Source: CAD feature listing. Evaluate the final solid. Frame: model axes, mm. Coordinates: 2 decimals unless noted, no trailing zeros. Write each loop counter-clockwise with the first axis right and the second up, starting at its lowest first coordinate (ties: lowest second). Pieces come first, ordered by that corner, then holes. Notation, with made-up numbers: (66.25, -9) -> (117.25, -9) arc R12 cw to (117.25, 13) -> close; hole circle Ø8 at (10.25, 62). An arc over 180 degrees is marked (long way). Write item = value, one per line.
from build123d import *

# Parameters (mm, degrees)
SKETCH1_R           = 1.5
BOSS_EXTRUDE1_DEPTH = 2
CHAMFER1_SIZE       = 0.25


with BuildPart() as part:
    # Sketch1 → Boss-Extrude1 (new body)
    with BuildSketch(Plane(origin=(0, 0, 0), x_dir=(1, 0, 0), z_dir=(0, 1, 0))):
        Polygon((0, -3.464101615), (3, -1.732050808), (3, 1.732050808), (0, 3.464101615), (-3, 1.732050808), (-3, -1.732050808), align=None)
        Circle(SKETCH1_R, mode=Mode.SUBTRACT)
    extrude(amount=BOSS_EXTRUDE1_DEPTH)

    # Chamfer1
    chamfer1_edges = [part.edges().sort_by_distance(p)[0] for p in [
        (3, 2, 0),
        (1.5, 2, -2.598076211),
        (-1.5, 0, 0),
        (-1.5, 2, 0),
        (-1.5, 2, -2.598076211),
        (-3, 2, 0),
        (-1.5, 2, 2.598076211),
        (-3, 0, 0),
        (-1.5, 0, -2.598076211),
        (1.5, 0, -2.598076211),
        (3, 0, 0),
        (1.5, 0, 2.598076211),
        (-1.5, 0, 2.598076211),
        (1.5, 2, 2.598076211),
    ]]
    chamfer(chamfer1_edges, length=CHAMFER1_SIZE)


solid = part.part
1) First-contact query: pin 1 Ø2 at (x, z) = (0.5, 0.5) entering from -Y; pin 2 Ø1.8 at (x, z) = (0, 0) entering from -Y. Flat tips, straight axial feed; report the tip coordinate or a pass-through.
Answer block:
pin_1 = 0.04
pin_2 = through
2) Cut plane C-C, the plane x = -2.25. Output: boundary loops of the cut face in (y, z), and give its area (3 significant figures).
Answer block:
outline = (0, -1.88) -> (0.25, -2.17) -> (1.75, -2.17) -> (2, -1.88) -> (2, 1.88) -> (1.75, 2.17) -> (0.25, 2.17) -> (0, 1.88) -> close
area = 8.52 mm2
3) Material intervals for probe 1 along X at (y, z) = (0.85, 0); probe 2 along X at (y, z) = (0.45, 1.25); probe 3 along Z at (x, y) = (1.25, 1.1), sorted ascending. Write a range as [from, to].
Answer block:
probe_1 = [-3, -1.5], [1.5, 3]
probe_2 = [-3, -0.83], [0.83, 3]
probe_3 = [-2.74, -0.83], [0.83, 2.74]
4) Cut plane A-A, the plane y = 1.2. Output: boundary loops of the cut face in (x, z), and give its area (3 significant figures).
Answer block:
outline = (-3, -1.73) -> (0, -3.46) -> (3, -1.73) -> (3, 1.73) -> (0, 3.46) -> (-3, 1.73) -> close; hole circle Ø3 at (0, 0)
area = 24.1 mm2
5) Cut plane D-D, the plane y = 1.9. Output: boundary loops of the cut face in (x, z), and give its area (3 significant figures).
Answer block:
outline = (-2.85, -1.65) -> (0, -3.29) -> (2.85, -1.65) -> (2.85, 1.65) -> (0, 3.29) -> (-2.85, 1.65) -> close; hole circle Ø3.3 at (0, 0)
area = 19.6 mm2
6) Pull-direction query (X, two-part tool) for faces 1 (the cylindrical face through (-1.5, 0.99, -0.07)), 2 (the flat face through (1.416, 0.123, 2.5)), 3 (the flat face through (-1.416, 0.123, -2.5)), 4 (the flat face through (-1.3, 2, 1.4)); classes: +X half, -X half, draft (parallel to the pull), parting line (faces both ways), or undercut.
Answer block:
face_1 = undercut
face_2 = +X half
face_3 = -X half
face_4 = draft
7) Cut plane B-B, the plane z = -2. Output: boundary loops of the cut face in (x, y).
Answer block:
outline = (-2.54, 0.25) -> (-2.04, 0) -> (2.04, 0) -> (2.54, 0.25) -> (2.54, 1.75) -> (2.04, 2) -> (-2.04, 2) -> (-2.54, 1.75) -> close
